Design review of the part shown in the three views and the two pictorial views. Dimensions are in mm from the part's minimum x, y and z. A direction names the side the tool comes from. Round coordinates to 2 decimals unless told otherwise and drop trailing zeros. Loops run counter-clockwise (first coordinate to the right, second up) from the corner with the lowest first, then second, coordinate; pieces in that order, holes last. Notation, with made-up numbers: M 14.5,76.25 L 25.5,76.25 A22 ccw 25.5,83.25 Z; hole C 37,-10.75 d11. An arc over 180 degrees is marked long. Answer as CSV lines item,"result". Start each with the question number.
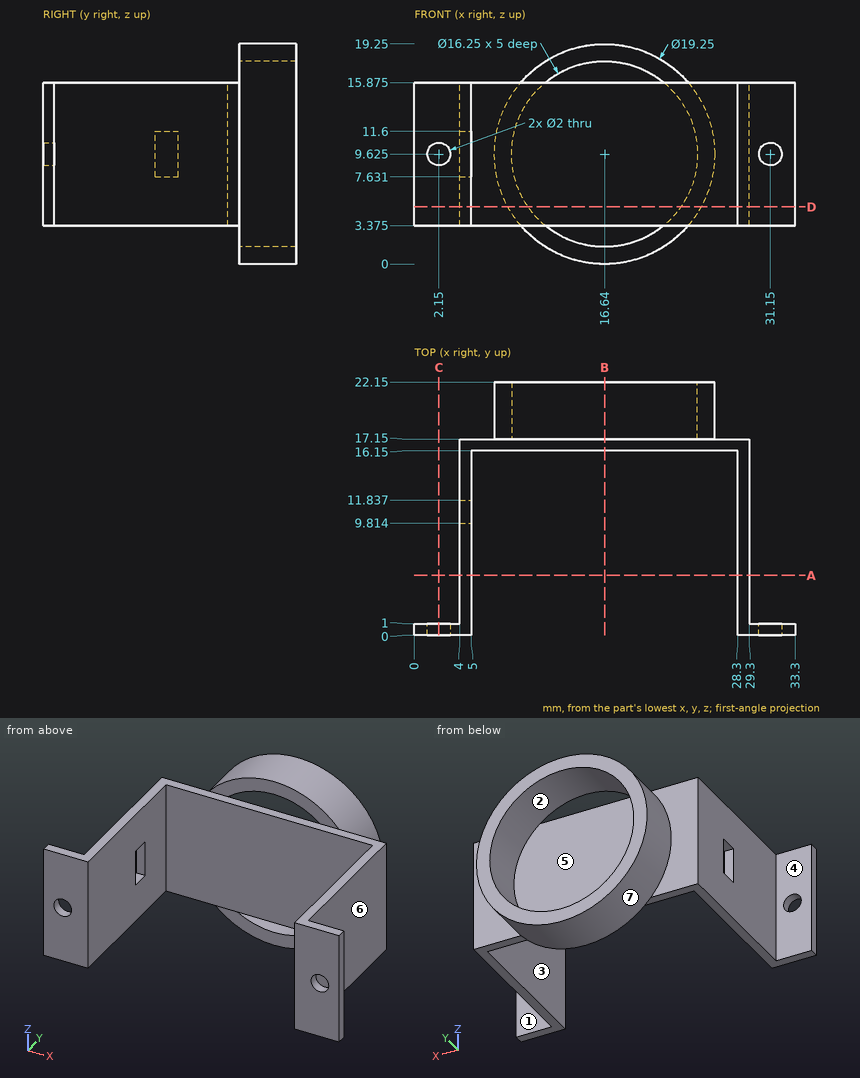
Item 1: Consider section C-C, the plane x = 2.15. Write out the cut boundary in (y, z) (1 decimal).
Item 2: Consider section A-A, the plane y = 5.25. Write out the cut boundary in (x, z) (1 decimal), then the cut area to 3 significant figures.
Item 3: Insertion check: pin 1 Ø3 at (x, y) = (25, 17) entering from -Z; pin 2 Ø10 at (x, z) = (13, 9) entering from -Y; pin 3 Ø1.1 at (x, z) = (4.5, 10) entering from +Y. Each pin has a flat end and moves straight along its axis. Give the tip position at first contact, or say it passes through.
Item 4: To check wall thickness, follow line 1 (Z direction, x = 2.15, y = 0.65) (1 decimal); line 2 (X direction, y = 12.25, z = 10.25); line 3 (Y direction, x = 16.5, z = 10.75). State the ranges of each line that lie inside material, in increasing order.
Item 5: Consider section D-D, the plane z = 5. Write out the cut boundary in (x, y).
Item 6: Consider section B-B, the plane x = 16.64. Count the separate pieces of the cut face and the enclosed holes in it, then the cut area to 3 significant figures.
Item 7: The part is to be moulded in two halves that separate along X. For the marked faces 5, 6 and 7, say which applies: +X half, -X half, draft (parallel to the pull), parting line (faces both ways), or undercut.
Item 8: Tool access review of the marked faces 1, 2, 3 and 4: name each direction out of +Z, -Z, +X, -X, +Y, -Y from which nothing blocks a thin tool from reaching the whole face with its end or side.
Found:
1,outline,"M 0,3.4 L 1,3.4 L 1,8.6 L 0,8.6 Z; M 0,10.6 L 1,10.6 L 1,15.9 L 0,15.9 Z"
2,outline,"M 4,3.4 L 5,3.4 L 5,15.9 L 4,15.9 Z; M 28.3,3.4 L 29.3,3.4 L 29.3,15.9 L 28.3,15.9 Z"
2,area,"25.0 mm^2"
3,pin 1,"stops at z = 2.88"
3,pin 2,"stops at y = 16.15"
3,pin 3,"stops at y = 17.15"
4,line 1,"z = 3.4 to 8.6, 10.6 to 15.9"
4,line 2,"x = 4 to 5, 28.3 to 29.3"
4,line 3,"y = 16.15 to 17.15"
5,outline,"M 0,0 L 5,0 L 5,16.15 L 28.3,16.15 L 28.3,0 L 33.3,0 L 33.3,1 L 29.3,1 L 29.3,17.15 L 25.08,17.15 L 25.08,22.15 L 23.32,22.15 L 23.32,17.15 L 9.96,17.15 L 9.96,22.15 L 8.2,22.15 L 8.2,17.15 L 4,17.15 L 4,1 L 0,1 Z"
6,separate pieces,"3"
6,enclosed holes,"0"
6,area,"27.5 mm^2"
7,face 5,"undercut"
7,face 6,"+X half"
7,face 7,"parting line"
8,face 1,"+Z, -Z, +X, +Y"
8,face 2,"+Y"
8,face 3,"+Z, -Z, -Y"
8,face 4,"+Z, -Z, -X, +Y"
